Autodesk Inventor part; units mm, degrees
ref_plane "YZ Plane" through (0, 0, 0) normal (1, 0, 0) x (0, 1, 0)
ref_plane "XZ Plane" through (0, 0, 0) normal (0, 1, 0) x (-1, 0, 0)
ref_plane "XY Plane" through (0, 0, 0) normal (0, 0, 1) x (1, 0, 0)
sketch "Эскиз1" plane through (0, 0, 0) normal (0, 1, 0) x (-1, 0, 0)
  line L0 (81.6842, 653.4737) -> (-198.3158, 653.4737)
  line L1 (-198.3158, 653.4737) -> (-198.3158, -122.5263)
  line L2 (-198.3158, -122.5263) -> (81.6842, -122.5263)
  line L3 (81.6842, -122.5263) -> (81.6842, 653.4737)
  point P0 (0, 0)
  dimension "d0" = 776
  dimension "d1" = 280
extrude "Выдавливание1" add sketch "Эскиз1" along normal blind 20
sketch "Эскиз3" plane through (-81.6842, 0, 653.4737) normal (0, 0, 1) x (1, 0, 0)
  line L0 (292, 31) -> (240, 31)
  line L1 (240, 31) -> (240, 9)
  line L2 (240, 9) -> (292, 9)
  line L3 (292, 9) -> (292, 31)
  line L4 (0, 0) -> (280, 0)
  line L5 (280, 0) -> (280, 20)
  line L6 (-1, 23) -> (40, 23)
  line L7 (40, 23) -> (40, 9)
  line L8 (40, 9) -> (-1, 9)
  line L9 (-1, 9) -> (-1, 23)
  line L10 (0, 0) -> (0, 20)
  point P0 (81.6842, 0)
  dimension "d4" = 9
  dimension "d5" = 40
  dimension "d6" = 9
  dimension "d7" = 40
extrude "Выдавливание2" cut sketch "Эскиз3" against normal blind 999
sketch "Эскиз4" plane through (-81.6842, 0, 653.4737) normal (0, 0, 1) x (1, 0, 0)
  point P0 (81.6842, 0)
sketch "Эскиз5" plane through (-81.6842, 0, 653.4737) normal (0, 0, 1) x (1, 0, 0)
  line L0 (280, 0) -> (280, 9)
  line L1 (280, 0) -> (0, 0)
  line L2 (0, 0) -> (0, 20)
  line L3 (0, 20) -> (280, 20)
  line L4 (280, 20) -> (280, 0)
  point P0 (81.6842, 0)
  dimension "d18" = 20
extrude "Выдавливание3" add sketch "Эскиз5" along normal mid plane 52
sketch "Эскиз6" plane through (198.3158, 0, -122.5263) normal (0, 0, -1) x (-1, 0, 0)
  line L0 (0, 0) -> (280, 0)
  line L1 (0, 20) -> (0, 9)
  line L2 (280, 0) -> (0, 0)
  line L3 (0, 0) -> (0, 20)
  line L4 (0, 20) -> (280, 20)
  line L5 (280, 20) -> (280, 0)
  point P0 (198.3158, 0)
  point P1 (0, 9)
extrude "Выдавливание4" add sketch "Эскиз6" along normal mid plane 52
sketch "Эскиз7" plane through (0, 20, 0) normal (0, 1, 0) x (1, 0, 0)
  line L0 (-81.6842, -627.4737) -> (198.3158, -627.4737)
  line L1 (198.3158, 96.5263) -> (-81.6842, 96.5263)
  line L2 (198.3158, 96.5263) -> (198.3158, -627.4737)
  line L3 (-149.6842, -265.4737) -> (289, -265.4737)
  line L4 (289, -265.4737) -> (289, -7.4737)
  line L5 (289, -7.4737) -> (-149.6842, -7.4737)
  line L6 (-149.6842, -7.4737) -> (-149.6842, -265.4737)
  line L7 (-149.6842, -265.4737) -> (289, -265.4737)
  line L8 (289, -265.4737) -> (289, -523.4737)
  line L9 (289, -523.4737) -> (-149.6842, -523.4737)
  line L10 (-149.6842, -523.4737) -> (-149.6842, -265.4737)
  point P0 (0, 0)
  dimension "d14" = 258
  dimension "d15" = 258
extrude "Выдавливание5" cut sketch "Эскиз7" against normal blind 1
properties part number "NizFlanecX_ax"
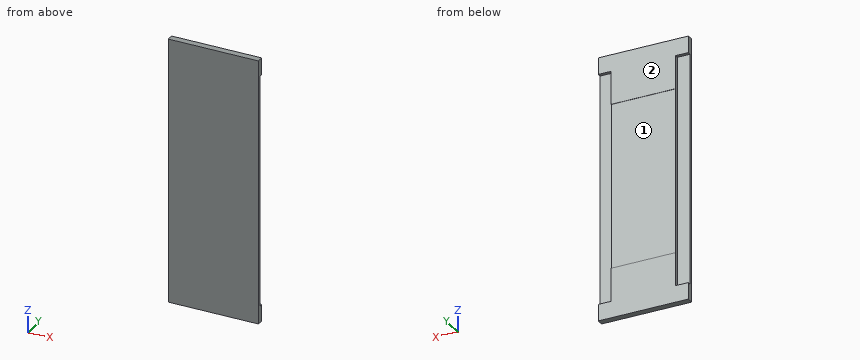
Build history of the part. All positions in model axes, mm. Face numbers are marked on the shaded views. Coordinates: 2 decimals unless noted, no trailing zeros. Order: outer loops, then holes, each group sorted by start corner. A loop starts at its lowest first (then second) coordinate and runs counter-clockwise, first axis right, second up. Notation, with made-up numbers: (67.5, 8.25) - (104.5, 8.25) arc R5 ccw to (104.5, 12.25) - close; hole circle Ø10 at (40, -32). An arc over 180 degrees is marked (long way). Put each result on its own line as item: value.
1. Saw through at C-C (y = 14). Write the cut outline in (x, z).
Answer sheet:
outline: (-81.68, -148.53) - (198.32, -148.53) - (198.32, -96.53) - (158.32, -96.53) - (158.32, 627.47) - (198.32, 627.47) - (198.32, 679.47) - (-81.68, 679.47) - (-81.68, 627.47) - (-41.68, 627.47) - (-41.68, -96.53) - (-81.68, -96.53) - close
2. Probe line 1 along Y through (x, z) = (20.5, 239); line 2 along X through (y, z) = (18.25, 151); line 3 along Z through (x, y) = (187, 10). List the from-to ranges inside material, lowest first. Write a range as [from, to].
Answer sheet:
line 1: y = [0, 19]
line 2: x = [-41.68, 158.32]
line 3: z = [-148.53, -96.53], [627.47, 679.47]
3. Saw through at B-B (x = -34). Write the cut outline in (y, z), and give its area (3 significant figures).
Answer sheet:
outline: (0, -148.53) - (20, -148.53) - (20, 7.47) - (19, 7.47) - (19, 523.47) - (20, 523.47) - (20, 679.47) - (0, 679.47) - close
area: 16,000 mm^2
4. Saw through at A-A (z = -22.5). Write the cut outline in (x, y), and give its area (3 significant figures).
Answer sheet:
outline: (-81.68, 0) - (198.32, 0) - (198.32, 9) - (158.32, 9) - (158.32, 20) - (-41.68, 20) - (-41.68, 9) - (-81.68, 9) - close
area: 4,720 mm^2
5. Drop flat-ended pins along their axis: P1, Ø10, axis at x = 1.5, z = 246, coming from the +Y side; P2, Ø9, axis at y = 16, z = 172.5, coming from the +X side; P3, Ø9, axis at y = 15, z = 351.5, coming from the -X side; P4, Ø4, axis at y = 10.5, z = 384, coming from the -X side. Give the stop position or say it passes through.
Answer sheet:
P1: stops at y = 19
P2: stops at x = 158.32
P3: stops at x = -41.68
P4: stops at x = -81.68
6. Pull direction Z, two halves, no side cores. Call the marked faces 1 and 2: pulls with the +Z half, pulls with the -Z half, needs draft (parallel to the pull), parting line crosses it, or undercut.
Answer sheet:
face 1: undercut
face 2: needs draft
